from build123d import *

# Parameters (mm, degrees)
SKETCH_1_R          = 22.5
SKETCH_1_R_2        = 10
EXTRUDE_1_DEPTH     = 6.5
SKETCH_2_R          = 2
CUT_EXTRUDE_1_DEPTH = 7.5
SKETCH_3_R          = 11
CUT_EXTRUDE_2_DEPTH = 5
CHAMFER_1_SIZE      = 2
CHAMFER_1_SIZE2     = 3.4


with BuildPart() as part:
    # 草图1 → 凸台-拉伸1 (new body)
    with BuildSketch(Plane(origin=(0, 0, 0), x_dir=(1, 0, 0), z_dir=(0, 1, 0))):
        Circle(SKETCH_1_R)
        Circle(SKETCH_1_R_2, mode=Mode.SUBTRACT)
    extrude(amount=EXTRUDE_1_DEPTH)

    # 草图2 → 切除-拉伸1 (cut, through all)
    with BuildSketch(Plane(origin=(0, 6.5, 0), x_dir=(1, 0, 0), z_dir=(0, 1, 0))):
        with Locations((0, 17.5)):
            Circle(SKETCH_2_R)
        with Locations((17.5, 0)):
            Circle(SKETCH_2_R)
        with Locations((0, -17.5)):
            Circle(SKETCH_2_R)
        with Locations((-17.5, 0)):
            Circle(SKETCH_2_R)
    extrude(amount=-CUT_EXTRUDE_1_DEPTH, mode=Mode.SUBTRACT)

    # 草图3 → 切除-拉伸2 (cut)
    with BuildSketch(Plane.XZ):
        Circle(SKETCH_3_R)
    extrude(amount=-CUT_EXTRUDE_2_DEPTH, mode=Mode.SUBTRACT)

    # 倒角1
    chamfer_1_edges = [part.edges().sort_by_distance(p)[0] for p in [
        (-2, 6.5, -17.5),
        (15.5, 6.5, 0),
        (-2, 6.5, 17.5),
        (-19.5, 6.5, 0),
    ]]
    chamfer_1_side = [part.faces().sort_by_distance(p)[0] for p in [
        (-21.863603897, 6.5, 0),
    ]]
    chamfer(chamfer_1_edges, length=CHAMFER_1_SIZE, length2=CHAMFER_1_SIZE2, reference=chamfer_1_side[0])


solid = part.part
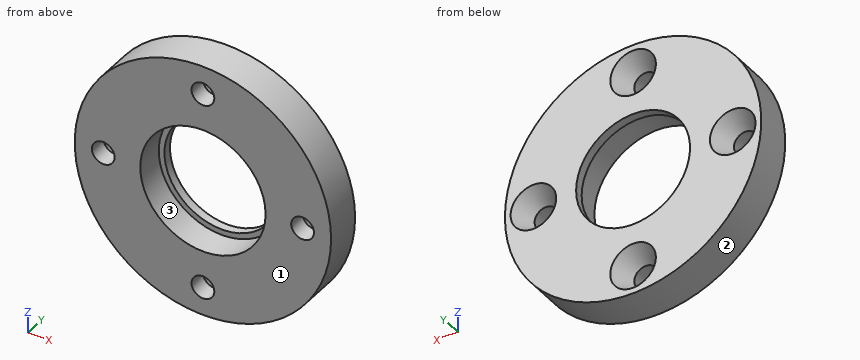
Work out the finished part from the listing and answer in its coordinate system (mm). Face numbers are marked on the shaded views. Coordinates: 2 decimals unless noted, no trailing zeros. Write each loop counter-clockwise with the first axis right and the second up, starting at its lowest first coordinate (ties: lowest second). Pieces come first, ordered by that corner, then holes. Notation, with made-up numbers: M -9,-17 L 44,-17 A14 ccw 44,8 Z; hole C 67.25,77 d2. An arc over 180 degrees is marked long. Use one line per item in the form item = value. Start each with the question number.
1. The part is cut by section D-D (z = 17.5). Give the vertices of the cut face in (x, y).
2. The part is cut by section C-C (x = 17.5). Give the vertices of the cut face in (y, z), plus the area to 3 significant figures.
3. Each of these flat-tipped pins is pushed along its axis until it touches: P1, Ø6.5, axis at x = 0, z = -17.5, coming from the +Y side (3 decimals); P2, Ø1, axis at y = 2, z = -14, coming from the -X side; P3, Ø2, axis at x = -12.5, y = 5, coming from the -Z side. Where does it stop, or does it pass through?
4. The part is cut by section A-A (z = 0). Give the vertices of the cut face in (x, y), plus the area to 3 significant figures.
5. The part is cut by section B-B (y = 2). Give the vertices of the cut face in (x, z), plus the area to 3 significant figures.
6. The mould has two halves that part along Z. Classify the marked faces 1, 2 and 3: released by +Z, released by -Z, zero draft, split by the parting line, or undercut.
7. Straight lines are drawn through the part: probe 1 along Z at (x, y) = (0, 1.35); probe 2 along Z at (x, y) = (0, 5.4); probe 3 along Y at (x, z) = (6, -8.5). For each, find the intervals that lie inside material, in ascending order. Write a range as from..to.
Evaluation:
q1.outline = M -14.14,0 L -2,0 L -2,3.1 L -4,6.5 L -14.14,6.5 Z; M 2,0 L 14.14,0 L 14.14,6.5 L 4,6.5 L 2,3.1 Z
q2.outline = M 0,-14.14 L 6.5,-14.14 L 6.5,-4 L 3.1,-2 L 0,-2 Z; M 0,2 L 3.1,2 L 6.5,4 L 6.5,14.14 L 0,14.14 Z
q2.area = 151 mm^2
q3.P1 = 5.225
q3.P2 = -18
q3.P3 = -19.34
q4.outline = M -22.5,0 L -19.5,0 L -19.5,3.1 L -21.5,6.5 L -22.5,6.5 Z; M -15.5,0 L -11,0 L -11,5 L -10,5 L -10,6.5 L -13.5,6.5 L -15.5,3.1 Z; M 10,5 L 11,5 L 11,0 L 15.5,0 L 15.5,3.1 L 13.5,6.5 L 10,6.5 Z; M 19.5,0 L 22.5,0 L 22.5,6.5 L 21.5,6.5 L 19.5,3.1 Z
q4.area = 86.9 mm^2
q5.outline = C 0,0 d45; hole C -17.5,0 d4; hole C 0,0 d22; hole C 0,-17.5 d4; hole C 0,17.5 d4; hole C 17.5,0 d4
q5.area = 1,160 mm^2
q6.face_1 = zero draft
q6.face_2 = split by the parting line
q6.face_3 = undercut
q7.probe_1 = -22.5..-19.5, -15.5..-11, 11..15.5, 19.5..22.5
q7.probe_2 = -22.5..-20.85, -14.15..-10, 10..14.15, 20.85..22.5
q7.probe_3 = 5..6.5
